Design review of the part built by this model. Coordinates are the model's own, in mm. Give positions to 0.01 mm unless a question says otherwise; leave off trailing zeros. Write each loop counter-clockwise with the first axis right and the second up, starting at its lowest first coordinate (ties: lowest second). Pieces come first, ordered by that corner, then holes.
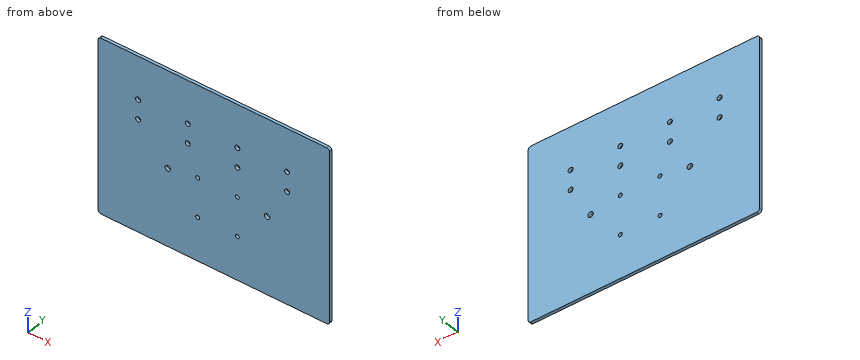
Autodesk Inventor part; units mm, degrees
ref_plane "YZ Plane" through (0, 0, 0) normal (1, 0, 0) x (0, 1, 0)
ref_plane "XZ Plane" through (0, 0, 0) normal (0, 1, 0) x (-1, 0, 0)
ref_plane "XY Plane" through (0, 0, 0) normal (0, 0, 1) x (1, 0, 0)
sketch "Sketch1" plane through (0, 0, 0) normal (0, 1, 0) x (-1, 0, 0)
  line L0 (232.1908, -176.5808) -> (232.1908, -3.7592)
  arc A0 (232.1908, -3.7592) -> (227.4316, 1) centre (227.4316, -3.7592) ccw
  line L1 (227.4316, 1) -> (0, 1)
  arc A1 (0, 1) -> (-4.7592, -3.7592) centre (0, -3.7592) ccw
  arc A2 (-4.7592, -176.5808) -> (0, -181.34) centre (0, -176.5808) ccw
  arc A3 (227.4316, -181.34) -> (232.1908, -176.5808) centre (227.4316, -176.5808) ccw
  circle A4 centre (130, -135) radius 2
  circle A5 centre (130, -95) radius 2
  circle A6 centre (90, -135) radius 2
  circle A7 centre (90, -95) radius 2
  circle A8 centre (160.0797, -100) radius 2.75
  circle A9 centre (60.0797, -100) radius 2.75
  circle A10 centre (90, -45) radius 2.5
  circle A11 centre (190, -45) radius 2.5
  circle A12 centre (190, -65) radius 2.5
  circle A13 centre (90, -65) radius 2.5
  circle A14 centre (140, -45) radius 2.5
  circle A15 centre (40, -45) radius 2.5
  circle A16 centre (140, -65) radius 2.5
  circle A17 centre (40, -65) radius 2.5
  line L2 (230.1908, -176.5808) -> (230.1908, -3.7592)
  arc A18 (230.1908, -3.7592) -> (227.4316, -1) centre (227.4316, -3.7592) ccw
  line L3 (227.4316, -1) -> (0, -1)
  arc A19 (0, -1) -> (-2.7592, -3.7592) centre (0, -3.7592) ccw
  arc A20 (-2.7592, -176.5808) -> (0, -179.34) centre (0, -176.5808) ccw
  arc A21 (227.4316, -179.34) -> (230.1908, -176.5808) centre (227.4316, -176.5808) ccw
  line L4 (-4.7592, -3.7592) -> (-4.7592, -176.5808)
  line L5 (-2.7592, -3.7592) -> (-2.7592, -176.5808)
  line L6 (0, -179.34) -> (227.4316, -179.34)
  line L7 (227.4316, -181.34) -> (0, -181.34)
  point P0 (0, 0)
  point P1 (230.1908, -3.7592)
  point P2 (0, -1)
  dimension "d0" = 2
  dimension "d1" = 2
  dimension "d2" = 2
  dimension "d3" = 2
  dimension "d5" = 2
  dimension "d7" = 2
  dimension "d8" = 227.4316
  dimension "d9" = 172.8216
  dimension "d10" = 4.7592
extrude "Extrusion1" add sketch "Sketch1" along normal blind 3 contours A21 L6 A20 L5 A19 L3 A18 L2
sketch "Sketch2" plane through (0, 3, 0) normal (0, 1, 0) x (1, 0, 0)
  line L0 (-232.1908, 176.5808) -> (-232.1908, 3.7592)
  arc A0 (-232.1908, 3.7592) -> (-227.4316, -1) centre (-227.4316, 3.7592) ccw
  line L1 (-227.4316, -1) -> (0, -1)
  arc A1 (0, -1) -> (4.7592, 3.7592) centre (0, 3.7592) ccw
  arc A2 (4.7592, 176.5808) -> (0, 181.34) centre (0, 176.5808) ccw
  arc A3 (-227.4316, 181.34) -> (-232.1908, 176.5808) centre (-227.4316, 176.5808) ccw
  circle A4 centre (-130, 135) radius 2
  circle A5 centre (-130, 95) radius 2
  circle A6 centre (-90, 135) radius 2
  circle A7 centre (-90, 95) radius 2
  circle A8 centre (-160.0797, 100) radius 2.75
  circle A9 centre (-60.0797, 100) radius 2.75
  circle A10 centre (-90, 45) radius 2.5
  circle A11 centre (-190, 45) radius 2.5
  circle A12 centre (-190, 65) radius 2.5
  circle A13 centre (-90, 65) radius 2.5
  circle A14 centre (-140, 45) radius 2.5
  circle A15 centre (-40, 45) radius 2.5
  circle A16 centre (-140, 65) radius 2.5
  circle A17 centre (-40, 65) radius 2.5
  line L2 (-230.1908, 176.5808) -> (-230.1908, 3.7592)
  arc A18 (-230.1908, 3.7592) -> (-227.4316, 1) centre (-227.4316, 3.7592) ccw
  line L3 (-227.4316, 1) -> (0, 1)
  arc A19 (0, 1) -> (2.7592, 3.7592) centre (0, 3.7592) ccw
  arc A20 (2.7592, 176.5808) -> (0, 179.34) centre (0, 176.5808) ccw
  arc A21 (-227.4316, 179.34) -> (-230.1908, 176.5808) centre (-227.4316, 176.5808) ccw
  line L4 (4.7592, 3.7592) -> (4.7592, 176.5808)
  line L5 (2.7592, 3.7592) -> (2.7592, 176.5808)
  line L6 (0, 179.34) -> (-227.4316, 179.34)
  line L7 (-227.4316, 181.34) -> (0, 181.34)
  line L8 (0, 179.34) -> (-227.4316, 179.34)
  line L9 (-113.7158, 179.34) -> (-113.7158, 1)
  line L10 (-227.4316, 1) -> (0, 1)
  line L11 (-118.7158, 120.17) -> (-108.7158, 120.17)
  line L12 (-108.7158, 120.17) -> (-108.7158, 60.17)
  line L13 (-108.7158, 60.17) -> (-118.7158, 60.17)
  line L14 (-118.7158, 60.17) -> (-118.7158, 120.17)
  line L15 (-118.7158, 120.17) -> (-108.7158, 60.17) construction
  line L16 (-108.7158, 120.17) -> (-118.7158, 60.17) construction
  line L17 (-113.7158, 179.34) -> (-113.7158, 159.34)
  line L18 (2.7592, 139.34) -> (-230.1908, 139.34)
  line L19 (-230.1908, 139.34) -> (-230.1908, 179.34)
  line L20 (-230.1908, 179.34) -> (2.7592, 179.34)
  line L21 (2.7592, 179.34) -> (2.7592, 139.34)
  line L22 (2.7592, 139.34) -> (-230.1908, 179.34) construction
  line L23 (-230.1908, 139.34) -> (2.7592, 179.34) construction
  line L24 (-113.7158, 1) -> (-113.7158, 16)
  line L25 (-230.1908, 31) -> (2.7592, 31)
  line L26 (2.7592, 31) -> (2.7592, 1)
  line L27 (2.7592, 1) -> (-230.1908, 1)
  line L28 (-230.1908, 1) -> (-230.1908, 31)
  line L29 (-230.1908, 31) -> (2.7592, 1) construction
  line L30 (2.7592, 31) -> (-230.1908, 1) construction
  line L31 (-227.4316, 1) -> (0, 1)
  line L32 (-230.1908, 179.34) -> (-200.1908, 179.34)
  line L33 (-200.1908, 179.34) -> (-200.1908, 1)
  line L34 (-200.1908, 1) -> (-230.1908, 1)
  line L35 (-230.1908, 1) -> (-230.1908, 179.34)
  line L36 (2.7592, 1) -> (-27.2408, 1)
  line L37 (-27.2408, 1) -> (-27.2408, 179.34)
  line L38 (-27.2408, 179.34) -> (2.7592, 179.34)
  line L39 (2.7592, 179.34) -> (2.7592, 1)
  point P0 (230.1908, -176.5808)
  point P1 (230.1908, -3.7592)
  point P2 (227.4316, -1)
  point P3 (0, -1)
  point P4 (0, 0)
  point P5 (230.1908, -176.5808)
  point P6 (230.1908, -3.7592)
  point P7 (227.4316, -1)
  point P8 (0, -1)
  point P9 (-113.7158, 90.17)
  point P10 (-113.7158, 120.17)
  point P11 (-113.7158, 60.17)
  point P12 (-113.7158, 1)
  point P13 (0, 1)
  dimension "d22" = 2
  dimension "d23" = 2
  dimension "d24" = 2
  dimension "d25" = 2
  dimension "d26" = 2
  dimension "d27" = 2
  dimension "d28" = 227.4316
  dimension "d29" = 172.8216
  dimension "d30" = 4.7592
  dimension "d31" = 10
  dimension "d32" = 60
  dimension "d37" = 20
  dimension "d38" = 40
  dimension "d39" = 15
  dimension "d40" = 30
  dimension "d41" = 30
  dimension "d42" = 30
equation "\"d1\" = d0"
equation "\"d2\" = d0"
equation "\"d3\" = d0"
equation "\"d5\" = d0"
equation "\"d7\" = d0"
equation "\"d23\" = d22"
equation "\"d24\" = d22"
equation "\"d25\" = d22"
equation "\"d26\" = d22"
equation "\"d27\" = d22"
properties part number "EboxBottom"
(1) Consider section A-A, the plane x = -40. Give the boundary of the cut face in (y, z).
Resolved:
outline: (0, -179.34) - (3, -179.34) - (3, -67.5) - (0, -67.5) - close; (0, -62.5) - (3, -62.5) - (3, -47.5) - (0, -47.5) - close; (0, -42.5) - (3, -42.5) - (3, -1) - (0, -1) - close
(2) Consider section B-B, the plane z = -65. Give the boundary of the cut face in (x, y), then the cut area to 3 significant figures.
Resolved:
outline: (-230.19, 0) - (-192.5, 0) - (-192.5, 3) - (-230.19, 3) - close; (-187.5, 0) - (-142.5, 0) - (-142.5, 3) - (-187.5, 3) - close; (-137.5, 0) - (-92.5, 0) - (-92.5, 3) - (-137.5, 3) - close; (-87.5, 0) - (-42.5, 0) - (-42.5, 3) - (-87.5, 3) - close; (-37.5, 0) - (2.76, 0) - (2.76, 3) - (-37.5, 3) - close
area: 639 mm2
(3) To check wall thickness, follow L1, parallel to Z at x = -40, y = 1.95; L2, parallel to Z at x = -90, y = 0.7; L3, parallel to Z at x = -189, y = 1.55. State the ranges of each line that lie inside material, in increasing order.
Resolved:
L1: z = -179.34 to -67.5, -62.5 to -47.5, -42.5 to -1
L2: z = -179.34 to -137, -133 to -97, -93 to -67.5, -62.5 to -47.5, -42.5 to -1
L3: z = -179.34 to -67.29, -62.71 to -47.29, -42.71 to -1
